Design review of the part shown in the three views and the two pictorial views. Dimensions are in mm from the part's minimum x, y and z. Coordinates: 2 decimals unless noted, no trailing zeros. Write each loop counter-clockwise with the first axis right and the second up, starting at its lowest first coordinate (ties: lowest second). Pieces come first, ordered by that corner, then holes. Notation, with made-up numbers: (30.5, 76) - (81.5, 76) arc R19 cw to (81.5, 105) - close; hole circle Ø11 at (21.25, -7). An arc over 180 degrees is marked (long way). Write each question's results on one line, items separated by ' | '.
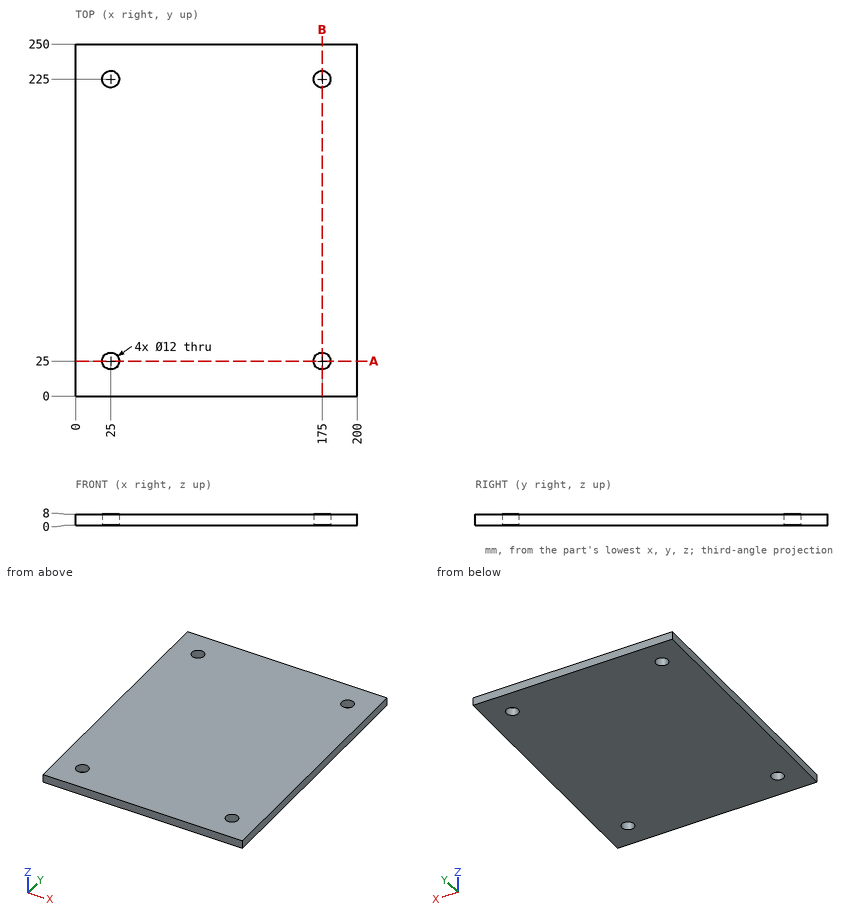
Q1. Take a section at A-A on y = 25. State the section outline as (x, z) points, plus the area to 3 significant figures.
Results found:
outline: (0, 0) - (19, 0) - (19, 8) - (0, 8) - close; (31, 0) - (169, 0) - (169, 8) - (31, 8) - close; (181, 0) - (200, 0) - (200, 8) - (181, 8) - close | area: 1,410 mm2
Q2. For pin 1 (7 mm diameter, centred on x = 175, y = 225, fed in from +Z), flat-tipped, find the tip position at first contact; note if it passes through.
Results found:
pin 1: through
Q3. Take a section at B-B on x = 175. State the section outline as (y, z) points.
Results found:
outline: (0, 0) - (19, 0) - (19, 8) - (0, 8) - close; (31, 0) - (219, 0) - (219, 8) - (31, 8) - close; (231, 0) - (250, 0) - (250, 8) - (231, 8) - close
Q4. Wall thickness on line 1 along Y through (x, z) = (175, 5.75); line 2 along X through (y, z) = (24, 7); line 3 along X through (y, z) = (220.5, 1.25): over which ranges is each line inside the solid? List them lowest first. Write a range as from..to.
Results found:
line 1: 0..19, 31..219, 231..250 | line 2: 0..19.08, 30.92..169.08, 180.92..200 | line 3: 0..21.03, 28.97..171.03, 178.97..200
